The model under review builds one solid part; all positions refer to its coordinate system, in mm. Face numbers are marked on the shaded views. Round coordinates to 2 decimals unless told otherwise and drop trailing zeros. Loops run counter-clockwise (first coordinate to the right, second up) from the corner with the lowest first, then second, coordinate; pieces in that order, holes last. Notation, with made-up numbers: M 88.25,84.5 L 104.25,84.5 A29 ccw 104.25,113.5 Z; hole C -40,67 d6. An arc over 180 degrees is marked long. Use a Markdown table: item, result. Add a question column.
```python
from build123d import *

# Parameters (mm, degrees)
SKETCH1_W             = 85
SKETCH1_H             = 30
TOP_SURFACE_DEPTH     = 10
SKETCH6_W             = 25
SKETCH6_H             = 5
TOP_SURFACE_CUT_DEPTH = 91.691785736
SKETCH8_R             = 0.64
BOSS_EXTRUDE2_DEPTH   = 1.3
LPATTERN2_COUNT       = 2
LPATTERN2_PITCH       = 83.7


with BuildPart() as part:
    # Sketch1 → Top surface (new body)
    with BuildSketch(Plane(origin=(0, 0, 0), x_dir=(1, 0, 0), z_dir=(0, 1, 0))):
        with Locations((42.5, 15)):
            Rectangle(SKETCH1_W, SKETCH1_H)
    extrude(amount=TOP_SURFACE_DEPTH)

    # Sketch6 → Top surface cut (cut, through all)
    with BuildSketch(Plane.ZY):
        with Locations((-12.5, 2.5)):
            Rectangle(SKETCH6_W, SKETCH6_H)
    extrude(amount=-TOP_SURFACE_CUT_DEPTH, mode=Mode.SUBTRACT)


with BuildPart() as part_1:
    # Body-Move/Copy1: moved
    add(part.part.moved(Location((0, 9.984827234, 0))))

    # Sketch8 → Boss-Extrude2 (add)
    with BuildSketch(Plane.ZY):
        with BuildLine():
            Line((-25.06, 9.984827234), (-29.94, 9.984827234))
            Line((-29.94, 9.984827234), (-29.94, 7.034827234))
            ThreePointArc((-29.94, 7.034827234), (-27.5, 4.594827234), (-25.06, 7.034827234))
            Line((-25.06, 7.034827234), (-25.06, 9.984827234))
        make_face()
        with Locations((-27.5, 7.034827234)):
            Circle(SKETCH8_R, mode=Mode.SUBTRACT)
    boss_extrude2 = extrude(amount=-BOSS_EXTRUDE2_DEPTH)

    # LPattern2: Boss-Extrude2 ×2
    with Locations(*[(i * LPATTERN2_PITCH, 0, 0) for i in range(1, LPATTERN2_COUNT)]):
        add(boss_extrude2)


solid = part_1.part
```
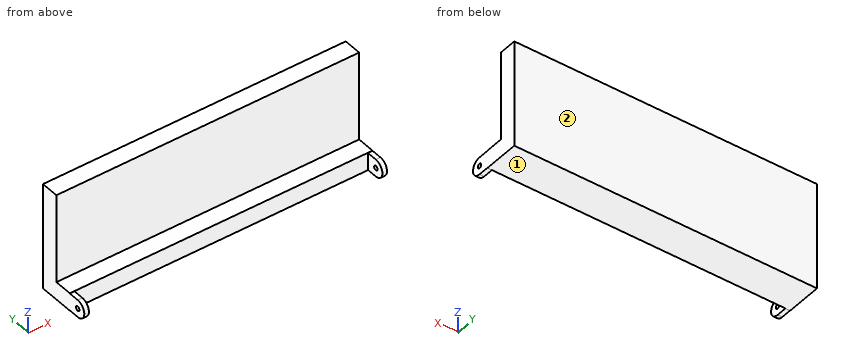
(1) Draft analysis for pull direction Z (two halves, no side actions). For the marked faces 1 and 2, state which applies: released by +Z, released by -Z, zero draft, split by the parting line, or undercut.
(2) Consider section B-B, the plane z = -16.75. Give the boundary of the cut face in (x, y), then the cut area to 3 significant figures.
(3) Insertion check: pin 1 Ø0.6 at (x, y) = (84, 8) entering from -Z; pin 2 Ø1.5 at (x, y) = (24, 12) entering from +Z; pin 3 Ø3 at (x, z) = (49, -6.5) entering from -Y. Each pin has a flat end and moves straight along its axis. Give the tip position at first contact, or say it passes through.
(4) Consider section C-C, the plane z = -26. Give the boundary of the cut face in (x, y).
(5) To check wall thickness, follow probe 1 along Y at (x, z) = (84.55, -27.5); probe 2 along Y at (x, z) = (54.5, -16.5); probe 3 along Z at (x, y) = (36, 14.25). State the ranges of each line that lie inside material, in increasing order.
(6) Consider section A-A, the plane x = 22.5. Give the boundary of the cut face in (y, z), then the cut area to 3 significant figures.
Found:
| question | item | result |
|---|---|---|
| 1 | face 1 | released by -Z |
| 1 | face 2 | zero draft |
| 2 | outline | M 0,14.98 L 85,14.98 L 85,19.98 L 0,19.98 Z |
| 2 | area | 425 mm^2 |
| 3 | pin 1 | stops at z = -29.94 |
| 3 | pin 2 | stops at z = -25 |
| 3 | pin 3 | stops at y = 14.98 |
| 4 | outline | M 0,5.11 L 1.3,5.11 L 1.3,9.98 L 83.7,9.98 L 83.7,5.11 L 85,5.11 L 85,19.98 L 0,19.98 Z |
| 5 | probe 1 | y = 4.59 to 6.39, 7.67 to 19.98 |
| 5 | probe 2 | y = 14.98 to 19.98 |
| 5 | probe 3 | z = -30 to -25 |
| 6 | outline | M 9.98,-30 L 19.98,-30 L 19.98,0 L 14.98,0 L 14.98,-25 L 9.98,-25 Z |
| 6 | area | 175 mm^2 |
